```python
from build123d import *

# Parameters (mm, degrees)
SKETCH015_W     = 27.500439
SKETCH015_H     = 13.55
SKETCH015_R     = 1.75
PAD007_DEPTH    = 24
SKETCH016_R     = 2.75
POCKET008_DEPTH = 8
SKETCH017_R     = 1.45
PAD008_DEPTH    = 1.6


with BuildPart() as part:
    # Sketch015 (on Face27 of Binder004) → Pad007 (new body)
    with BuildSketch(Plane.XZ.offset(-32.95)):
        with Locations((13.74978, -6.775)):
            Rectangle(SKETCH015_W, SKETCH015_H)
        with Locations((5.24978, -7.7)):
            Circle(SKETCH015_R, mode=Mode.SUBTRACT)
        with Locations((22.24978, -7.7)):
            Circle(SKETCH015_R, mode=Mode.SUBTRACT)
    extrude(amount=PAD007_DEPTH)

    # Sketch016 (on Face8 of Pad007) → Pocket008 (cut)
    with BuildSketch(Plane.XZ.offset(-8.95)):
        with Locations((5.24978, -7.7)):
            Circle(SKETCH016_R)
        with Locations((22.24978, -7.7)):
            Circle(SKETCH016_R)
    extrude(amount=-POCKET008_DEPTH, mode=Mode.SUBTRACT)

    # Sketch017 (on Face6 of Pocket008) → Pad008 (join)
    with BuildSketch(Plane.XY):
        with Locations((3, 13.5)):
            Circle(SKETCH017_R)
        with Locations((24.5, 13.5)):
            Circle(SKETCH017_R)
        with Locations((24.5, 30)):
            Circle(SKETCH017_R)
        with Locations((3, 30)):
            Circle(SKETCH017_R)
    extrude(amount=PAD008_DEPTH)


solid = part.part
```
Here's how the part is built. I have some questions about the finished solid (model axes, mm). A direction names the side the tool comes from. Coordinates: 2 decimals unless noted, no trailing zeros. Write each loop counter-clockwise with the first axis right and the second up, starting at its lowest first coordinate (ties: lowest second). Pieces come first, ordered by that corner, then holes. Notation, with made-up numbers: (-9, -39) -> (15, -39) arc R17 ccw to (15, -31) -> close; hole circle Ø10 at (27.5, 21.5). An arc over 180 degrees is marked (long way). Use a Markdown table: item, result. Add a question column.
(1) Please list where these lines run through material, in increasing order: line 1 (X direction, y = 29.75, z = -7.7); line 2 (Z direction, x = 5.25, y = 26.5); line 3 (X direction, y = 15, z = -8.25).
(2) If we section it at B-B, the plane y = 13.5: Write out the boundary of the cut face in (x, z), and give its area (3 significant figures).
(3) For faces 1 (the flat face through (24, 14, 1.6)), 2 (the flat face through (4, 16.95, -6)), 3 (the cylindrical face through (1.85, 12.62, 0.79)), which set-ups out of +Z, -Z, +X, -X, +Y, -Y let a thin tool reach every point of the face, with its end or its side?
(4) I'm going to push flat-ended pins straight in: P1, Ø5, axis at x = 5.25, z = -7.7, coming from the -Y side; P2, Ø6, axis at x = 22.5, z = -8, coming from the -Y side; P3, Ø7, axis at x = 20, y = 16, coming from the +Z side. Where does each tip first touch, or does it pass through?
(5) We'd pull the mould along Z, two halves only. Please class faces 4 (the flat face through (14, 21, -13.55)), 5 (the cylindrical face through (4.654, 12.894, -10.385)), 6 (the flat face through (21, 16.95, -6)), 7 (the flat face through (14, 8.95, -7)): +Z half, -Z half, draft (parallel to the pull), parting line (faces both ways), or undercut.
(6) If we section it at A-A, the plane z = -7.7: Write out the boundary of the cut face in (x, y), and give its area (3 significant figures).
(7) If we section it at C-C, the plane x = 5.75: Write out the boundary of the cut face in (y, z), and give its area (3 significant figures).
(8) If we section it at D-D, the plane y = 29: Write out the boundary of the cut face in (x, z), and give its area (3 significant figures).
Outcome:
| question | item | result |
|---|---|---|
| 1 | line 1 | x = 0 to 3.5, 7 to 20.5, 24 to 27.5 |
| 1 | line 2 | z = -13.55 to -9.45, -5.95 to 0 |
| 1 | line 3 | x = 0 to 2.56, 7.94 to 19.56, 24.94 to 27.5 |
| 2 | outline | (0, -13.55) -> (27.5, -13.55) -> (27.5, 0) -> (25.95, 0) -> (25.95, 1.6) -> (23.05, 1.6) -> (23.05, 0) -> (4.45, 0) -> (4.45, 1.6) -> (1.55, 1.6) -> (1.55, 0) -> (0, 0) -> close; hole circle Ø5.5 at (5.25, -7.7); hole circle Ø5.5 at (22.25, -7.7) |
| 2 | area | 334 mm^2 |
| 3 | face 1 | +Z, +X, -X, +Y, -Y |
| 3 | face 2 | -Y |
| 3 | face 3 | +Z |
| 4 | P1 | stops at y = 16.95 |
| 4 | P2 | stops at y = 8.95 |
| 4 | P3 | stops at z = 0 |
| 5 | face 4 | -Z half |
| 5 | face 5 | undercut |
| 5 | face 6 | undercut |
| 5 | face 7 | draft |
| 6 | outline | (0, 8.95) -> (2.5, 8.95) -> (2.5, 16.95) -> (3.5, 16.95) -> (3.5, 32.95) -> (0, 32.95) -> close; (7, 16.95) -> (8, 16.95) -> (8, 8.95) -> (19.5, 8.95) -> (19.5, 16.95) -> (20.5, 16.95) -> (20.5, 32.95) -> (7, 32.95) -> close; (24, 16.95) -> (25, 16.95) -> (25, 8.95) -> (27.5, 8.95) -> (27.5, 32.95) -> (24, 32.95) -> close |
| 6 | area | 460 mm^2 |
| 7 | outline | (8.95, -13.55) -> (32.95, -13.55) -> (32.95, -9.38) -> (16.95, -9.38) -> (16.95, -10.4) -> (8.95, -10.4) -> close; (8.95, -5) -> (16.95, -5) -> (16.95, -6.02) -> (32.95, -6.02) -> (32.95, 0) -> (8.95, 0) -> close |
| 7 | area | 228 mm^2 |
| 8 | outline | (0, -13.55) -> (27.5, -13.55) -> (27.5, 0) -> (25.55, 0) -> (25.55, 1.6) -> (23.45, 1.6) -> (23.45, 0) -> (4.05, 0) -> (4.05, 1.6) -> (1.95, 1.6) -> (1.95, 0) -> (0, 0) -> close; hole circle Ø3.5 at (5.25, -7.7); hole circle Ø3.5 at (22.25, -7.7) |
| 8 | area | 360 mm^2 |
